For this review, take the finished solid that the model builds, in its own axes (mm). A direction names the side the tool comes from. Coordinates: 2 decimals unless noted, no trailing zeros. Loops run counter-clockwise (first coordinate to the right, second up) from the corner with the lowest first, then second, coordinate; pieces in that order, holes last. Notation, with made-up numbers: M 24,-30.5 L 65,-30.5 A20 ccw 65,7.5 Z; hole C 5.5,-3.75 d4. An arc over 180 degrees is marked long. Answer as a JSON object with one key per item and string values. Group by question number.
Item 1: Add section A-A (z = 224.5). State the section outline as (x, y) points, then the cut area to 3 significant figures.
Item 2: Add section B-B (z = 132.5). State the section outline as (x, y) points, then the cut area to 3 significant figures.
Item 3: Insertion check: pin 1 (3 mm diameter, centred on y = 7, z = 205.5, fed in from -X); pin 2 (1.5 mm diameter, centred on x = 10.5, y = 3, fed in from -Z). Each pin has a flat end and moves straight along its axis. Give the tip position at first contact, or say it passes through.
Item 4: Tool access review of faces 5 (the face through (3, 8, 220)), 6 (the face through (11, 5, 250)), 7 (the face through (10.18, 0.35, 234.79)): name each direction out of +Z, -Z, +X, -X, +Y, -Y from which nothing blocks a thin tool from reaching the whole face with its end or side.
Item 5: Mouldability with a two-part tool opening along X and no side actions: class faces 1 (the face through (4.143, 5.07, 7.699)), 2 (the face through (5.5, 7.33, 235.21)), 3 (the face through (3, 2, 220)), 4 (the face through (16.99, 5.07, 2.85)) as +X half, -X half, draft (parallel to the pull), parting line (faces both ways), or undercut.
Item 6: Wall thickness on L1, parallel to X at y = 3, z = 9; L2, parallel to Z at x = 10.25, y = 1.5; L3, parallel to X at y = 1.25, z = 124.5: over which ranges is each line inside the solid? List them lowest first. Write a range as from..to.
from build123d import *

# Parameters (mm, degrees)
SKETCH2_W           = 20
SKETCH2_H           = 10
BOSS_EXTRUDE1_DEPTH = 250
SKETCH3_R           = 6
CUT_EXTRUDE1_DEPTH  = 30
FILLET1_R           = 10
FILLET3_R           = 10
SKETCH4_W           = 30
SKETCH4_H           = 10
BOSS_EXTRUDE2_DEPTH = 2.5
CUT_EXTRUDE2_DEPTH  = 30
FILLET4_R           = 5
FILLET5_R           = 10


with BuildPart() as part:
    # Sketch2 → Boss-Extrude1 (new body)
    with BuildSketch(Plane.XY):
        with Locations((10, 5)):
            Rectangle(SKETCH2_W, SKETCH2_H)
    extrude(amount=BOSS_EXTRUDE1_DEPTH)

    # Sketch3 → Cut-Extrude1 (cut)
    with BuildSketch(Plane(origin=(0, 10, 0), x_dir=(1, 0, 0), z_dir=(0, 1, 0))):
        with Locations(Location((10, -9, 0), (0, 0, 270))):
            Circle(SKETCH3_R)
    extrude(amount=-CUT_EXTRUDE1_DEPTH, mode=Mode.SUBTRACT)

    # Fillet1
    fillet1_edges = [part.edges().sort_by_distance(p)[0] for p in [
        (20, 5, 0),
    ]]
    fillet(fillet1_edges, radius=FILLET1_R)

    # Fillet3
    fillet3_edges = [part.edges().sort_by_distance(p)[0] for p in [
        (0, 5, 0),
    ]]
    fillet(fillet3_edges, radius=FILLET3_R - 0.0001)  # a hair under: the kernel refuses the full size

    # Sketch4 → Boss-Extrude2 (add)
    with BuildSketch(Plane.ZY):
        with Locations((235, 5)):
            Rectangle(SKETCH4_W, SKETCH4_H)
    extrude(amount=BOSS_EXTRUDE2_DEPTH)

    # Sketch5 → Cut-Extrude2 (cut)
    with BuildSketch(Plane.XY.offset(250)):
        Polygon((-2.5, 10), (-2.5, 5), (-0.5, 5.069841539), (2.5, 5.598822481), (10.123063076, 10), align=None)
        Polygon((-0.5, 4.930158461), (-2.5, 5), (-2.5, 0), (10.123063076, 0), (2.5, 4.401177519), align=None)
    extrude(amount=-CUT_EXTRUDE2_DEPTH, mode=Mode.SUBTRACT)

    # Fillet4
    fillet4_edges = [part.edges().sort_by_distance(p)[0] for p in [
        (2.5, 5.598822481, 235),
        (2.5, 4.401177519, 235),
    ]]
    fillet(fillet4_edges, radius=FILLET4_R)

    # Fillet5
    fillet5_edges = [part.edges().sort_by_distance(p)[0] for p in [
        (10.123063076, 10, 235),
        (10.123063076, 0, 235),
    ]]
    fillet(fillet5_edges, radius=FILLET5_R)


solid = part.part
From the geometry:
{
 "1": {"outline": "M -2.5,5 L -0.5,4.93 L 1.63,4.55 A5 cw 3.26,3.96 L 7.8,1.34 A10 ccw 12.8,0 L 20,0 L 20,10 L 12.8,10 A10 ccw 7.8,8.66 L 3.26,6.04 A5 cw 1.63,5.45 L -0.5,5.07 Z", "area": "142 mm²"},
 "2": {"outline": "M 0,0 L 20,0 L 20,10 L 0,10 Z", "area": "200 mm²"},
 "3": {"pin 1": "stops at x = 0", "pin 2": "stops at z = 0"},
 "4": {"face 5": "+Z, -X, +Y", "face 6": "+Z, +X, -X, +Y, -Y", "face 7": "+Z, -X, -Y"},
 "5": {"face 1": "undercut", "face 2": "-X half", "face 3": "draft", "face 4": "+X half"},
 "6": {"L1": "x = 0.05..4, 16..19.95", "L2": "z = 0..3.01, 14.99..250", "L3": "x = 0..20"}
}
